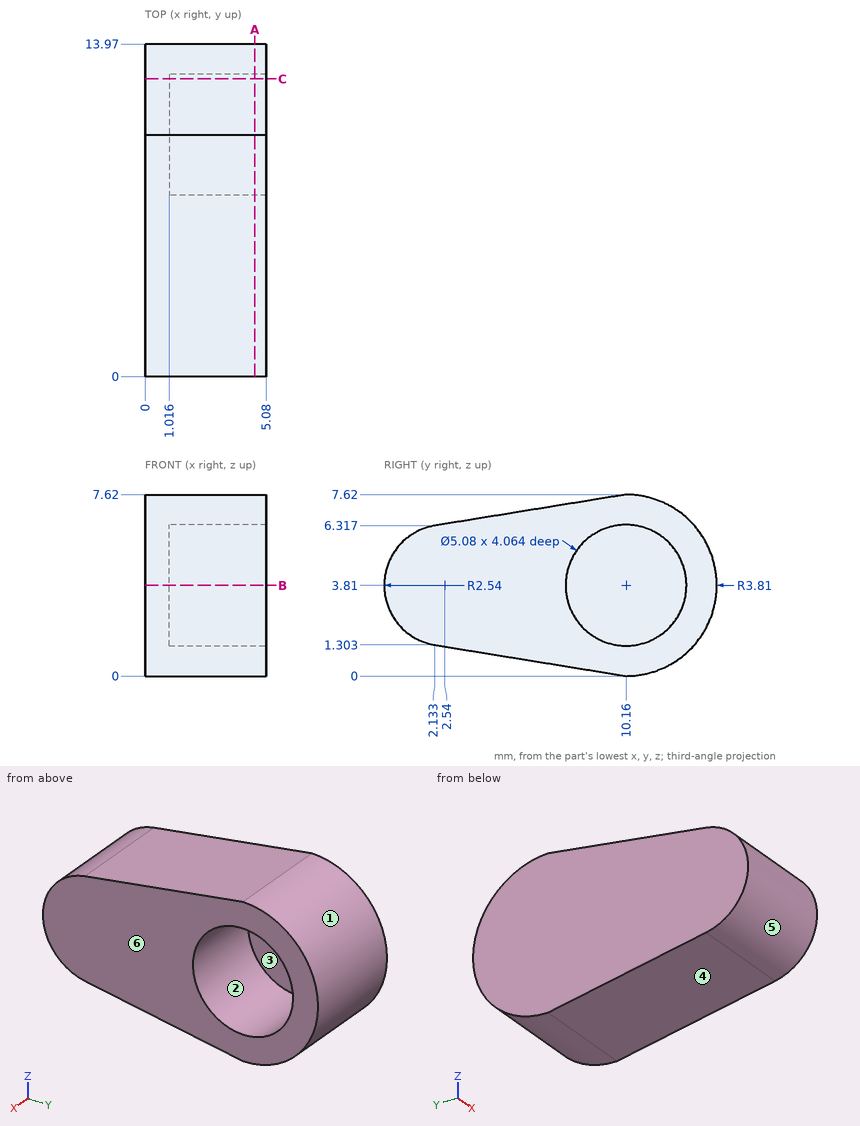
Can you work these out from the drawing? Everything is in mm from the part's minimum corner. A direction names the side the tool comes from. Round coordinates to 2 decimals unless told otherwise and drop trailing zeros. Loops run counter-clockwise (first coordinate to the right, second up) from the corner with the lowest first, then second, coordinate; pieces in that order, holes last. Notation, with made-up numbers: M 49,31.5 L 71,31.5 A21 ccw 71,61.5 Z; hole C 68,-13 d1. An arc over 180 degrees is marked long. Answer in a Markdown table with one row per item.
1. If we section it at A-A, the plane x = 4.6: Please give me the cut outline in (y, z), plus the area to 3 significant figures.
Established:
| item | result |
|---|---|
| outline | M 2.13,1.3 L 10.16,0 A3.81 ccw 10.16,7.62 L 2.13,6.32 A2.54 ccw Z; hole C 10.16,3.81 d5.08 |
| area | 61.3 mm² |
2. Thinking about a two-plate mould opening in Z: for the marked faces 3, 4, 5 and 6, which applies, pulls with the +Z half, pulls with the -Z half, needs draft (parallel to the pull), parting line crosses it, or undercut?
Established:
| item | result |
|---|---|
| face 3 | undercut |
| face 4 | pulls with the -Z half |
| face 5 | parting line crosses it |
| face 6 | needs draft |
3. On a 3-axis mill with a long thin cutter (end or side, diameter ignored), from which of +Z, -Z, +X, -X, +Y, -Y can I reach the whole of each face in a straight line? I mean the marked faces 1 and 2. Say none if no direction works.
Established:
| item | result |
|---|---|
| face 1 | +X, -X, +Y |
| face 2 | +X |
4. If we section it at C-C, the plane y = 12.5: Please give me the cut outline in (x, z).
Established:
| item | result |
|---|---|
| outline | M 0,0.8 L 5.08,0.8 L 5.08,2.82 L 1.02,2.82 L 1.02,4.8 L 5.08,4.8 L 5.08,6.82 L 0,6.82 Z |
5. Please list where these lines run through material, in increasing order: line 1 (Y direction, x = 1.65, z = 3.25); line 2 (X direction, y = 12, z = 2.25); line 3 (Y direction, x = 2.05, z = 2.25) (1 decimal). Write a range as from..to.
Established:
| item | result |
|---|---|
| line 1 | 0.06..7.68, 12.64..13.93 |
| line 2 | 0..1.02 |
| line 3 | 0.5..8.2, 12.2..13.6 |
6. If we section it at B-B, the plane z = 3.81: Please give me the cut outline in (x, y).
Established:
| item | result |
|---|---|
| outline | M 0,0 L 5.08,0 L 5.08,7.62 L 1.02,7.62 L 1.02,12.7 L 5.08,12.7 L 5.08,13.97 L 0,13.97 Z |
